from build123d import *

# Parameters (mm, degrees)
SKETCH1_W           = 100
SKETCH1_H           = 152
BOSS_EXTRUDE1_DEPTH = 34
SKETCH2_W           = 100
SKETCH2_H           = 145
CUT_EXTRUDE1_DEPTH  = 30
SKETCH3_W           = 7
SKETCH3_H           = 15
CUT_EXTRUDE2_DEPTH  = 158.101877774
SKETCH4_W           = 20.7
SKETCH4_H           = 145
CUT_EXTRUDE3_DEPTH  = 96.791440119
SKETCH5_W           = 25.4
SKETCH5_H           = 25.4
CUT_EXTRUDE4_DEPTH  = 96.791440119
SKETCH7_R           = 1.5
CUT_EXTRUDE5_DEPTH  = 96.791440119
SKETCH8_W           = 5
SKETCH8_H           = 12
CUT_EXTRUDE6_DEPTH  = 96.791440119


with BuildPart() as part:
    # Sketch1 → Boss-Extrude1 (new body)
    with BuildSketch(Plane(origin=(0, 0, 0), x_dir=(1, 0, 0), z_dir=(0, 1, 0))):
        Rectangle(SKETCH1_W, SKETCH1_H)
    extrude(amount=BOSS_EXTRUDE1_DEPTH)

    # Sketch2 → Cut-Extrude1 (cut)
    with BuildSketch(Plane(origin=(0, 34, 0), x_dir=(1, 0, 0), z_dir=(0, 1, 0))):
        with Locations((0, -3.5)):
            Rectangle(SKETCH2_W, SKETCH2_H)
    extrude(amount=-CUT_EXTRUDE1_DEPTH, mode=Mode.SUBTRACT)

    # Sketch3 → Cut-Extrude2 (cut, through all)
    with BuildSketch(Plane.XY.offset(-69)):
        with Locations((-39.9, 19)):
            Rectangle(SKETCH3_W, SKETCH3_H)
        with Locations((39.9, 19)):
            Rectangle(SKETCH3_W, SKETCH3_H)
    extrude(amount=-CUT_EXTRUDE2_DEPTH, mode=Mode.SUBTRACT)

    # Sketch4 → Cut-Extrude3 (cut, through all)
    with BuildSketch(Plane(origin=(0, 4, 0), x_dir=(1, 0, 0), z_dir=(0, 1, 0))):
        with Locations((-39.65, -3.5)):
            Rectangle(SKETCH4_W, SKETCH4_H)
        with Locations((39.65, -3.5)):
            Rectangle(SKETCH4_W, SKETCH4_H)
    extrude(amount=-CUT_EXTRUDE3_DEPTH, mode=Mode.SUBTRACT)

    # Sketch5 → Cut-Extrude4 (cut, through all)
    with BuildSketch(Plane(origin=(0, 4, 0), x_dir=(1, 0, 0), z_dir=(0, 1, 0))):
        with Locations((0, -53.7)):
            Rectangle(SKETCH5_W, SKETCH5_H)
    extrude(amount=-CUT_EXTRUDE4_DEPTH, mode=Mode.SUBTRACT)

    # Sketch7 → Cut-Extrude5 (cut, through all)
    with BuildSketch(Plane(origin=(0, 4, 0), x_dir=(1, 0, 0), z_dir=(0, 1, 0))):
        with Locations(Location((-10.3, -38.2, 0), (0, 0, 270))):
            Circle(SKETCH7_R)
        with Locations(Location((10.3, -38.2, 0), (0, 0, 270))):
            Circle(SKETCH7_R)
        with Locations(Location((10.3, -69.2, 0), (0, 0, 270))):
            Circle(SKETCH7_R)
        with Locations(Location((-10.3, -69.2, 0), (0, 0, 270))):
            Circle(SKETCH7_R)
    extrude(amount=-CUT_EXTRUDE5_DEPTH, mode=Mode.SUBTRACT)

    # Sketch8 → Cut-Extrude6 (cut, through all)
    with BuildSketch(Plane(origin=(0, 4, 0), x_dir=(1, 0, 0), z_dir=(0, 1, 0))):
        with Locations((15.2, -60.4)):
            Rectangle(SKETCH8_W, SKETCH8_H)
    extrude(amount=-CUT_EXTRUDE6_DEPTH, mode=Mode.SUBTRACT)


solid = part.part
Build history of the part. All positions in model axes, mm. A direction names the side the tool comes from. Coordinates: 2 decimals unless noted, no trailing zeros. Order: outer loops, then holes, each group sorted by start corner. A loop starts at its lowest first (then second) coordinate and runs counter-clockwise, first axis right, second up. Notation, with made-up numbers: (-36.5, 31) - (-19.5, 31) arc R26 ccw to (-19.5, 51) - close; hole circle Ø3 at (37, 19). An arc over 180 degrees is marked (long way). Write each question's results on one line, items separated by ' | '. Start each with the question number.
Item 1: Band-saw the part on A-A on z = 69.2. Write the cut outline in (x, y), and give its area (3 significant figures).
Item 2: Mould opens along X. For faces 1 (the face through (15, 2, 54.4)), 2 (the face through (40, 11.5, -72)), 3 (the face through (-50, 17, -72)), 4 (the face through (0, 4, 2)) say: released by +X, released by -X, zero draft, split by the parting line, or undercut.
Item 3: Band-saw the part on B-B on x = 3.5. Write the cut outline in (y, z), and give its area (3 significant figures).
Item 4: Tool access for faces 5 (the face through (17.7, 2, 60)), 6 (the face through (-36.4, 19, -72)), 7 (the face through (-1, 17, -76)), 8 (the face through (-29.3, 2, 5)): list every direction of +Z, -Z, +X, -X, +Y, -Y with a clear straight run to the whole face (end or side of a thin tool).
Item 5: Flat gauge pins, fed straight in: pin 1 (3 mm diameter, centred on y = 2.5, z = 33, fed in from +X); pin 2 (4 mm diameter, centred on y = 5.5, z = 43, fed in from -X); pin 3 (8 mm diameter, centred on x = 18, y = 18, fed in from +Z). Where does each tip first touch, or does it go through?
Item 6: Band-saw the part on D-D on x = 25.5. Write the cut outline in (y, z), and give its area (3 significant figures).
Item 7: Wall check: probe 1 along Z at (x, y) = (10, 1); probe 2 along X at (y, z) = (2.9, 69.2); probe 3 along Z at (x, y) = (26.5, 4.5). Give the ranges that are in metal, low to high. Write a range as [from, to].
Item 8: Band-saw the part on C-C on y = 22. Write the cut outline in (x, z), and give its area (3 significant figures).
Numbers:
1) outline: (-29.3, 0) - (-11.8, 0) - (-11.8, 4) - (-29.3, 4) - close; (-8.8, 0) - (8.8, 0) - (8.8, 4) - (-8.8, 4) - close; (11.8, 0) - (29.3, 0) - (29.3, 4) - (11.8, 4) - close | area: 210 mm^2
2) face 1: undercut | face 2: undercut | face 3: released by -X | face 4: zero draft
3) outline: (0, -76) - (34, -76) - (34, -69) - (4, -69) - (4, 41) - (0, 41) - close; (0, 66.4) - (4, 66.4) - (4, 76) - (0, 76) - close | area: 716 mm^2
4) face 5: +Y, -Y | face 6: +Z, -Z | face 7: -Z, +X, -X, +Y, -Y | face 8: +Z, -X, +Y, -Y
5) pin 1: x = 29.3 | pin 2: x = -29.3 | pin 3: z = -69
6) outline: (0, -76) - (34, -76) - (34, -69) - (4, -69) - (4, 76) - (0, 76) - close | area: 818 mm^2
7) probe 1: [-76, 36.73], [39.67, 41], [66.4, 67.73], [70.67, 76] | probe 2: [-29.3, -11.8], [-8.8, 8.8], [11.8, 29.3] | probe 3: [-76, -69]
8) outline: (-50, -76) - (-43.4, -76) - (-43.4, -69) - (-50, -69) - close; (-36.4, -76) - (36.4, -76) - (36.4, -69) - (-36.4, -69) - close; (43.4, -76) - (50, -76) - (50, -69) - (43.4, -69) - close | area: 602 mm^2
